Geometry: final body of the model. Coordinates: model frame, mm. Face numbers are marked on the shaded views. Round coordinates to 2 decimals unless told otherwise and drop trailing zeros. Loops run counter-clockwise (first coordinate to the right, second up) from the corner with the lowest first, then second, coordinate; pieces in that order, holes last. Notation, with made-up numbers: (14.25, 15) - (38.25, 15) arc R19 ccw to (38.25, 46) - close; hole circle Ø9 at (20, -3.75). An arc over 180 degrees is marked (long way). Answer in a Markdown table with one row per item. Add a question column.
from build123d import *

# Parameters (mm, degrees)
SKETCH_1_R          = 11
SKETCH_1_R_2        = 9.5
EXTRUDE_1_DEPTH     = 82
SKETCH_4_R          = 10
CUT_EXTRUDE_2_DEPTH = 2
CUT_EXTRUDE_START   = -2
SKETCH_5_R          = 10
CUT_EXTRUDE_3_DEPTH = 2
SKETCH_6_R          = 11.5
SKETCH_6_R_2        = 10.5
CUT_EXTRUDE_4_DEPTH = 0.5
SKETCH_7_R          = 11.5
SKETCH_7_R_2        = 10.5
CUT_EXTRUDE_5_DEPTH = 0.5


with BuildPart() as part:
    # Эскиз1 → Бобышка-Вытянуть1 (new body)
    with BuildSketch(Plane.XY):
        Circle(SKETCH_1_R)
        Circle(SKETCH_1_R_2, mode=Mode.SUBTRACT)
    extrude(amount=EXTRUDE_1_DEPTH)

    # Эскиз4 → Вырез-Вытянуть2 (cut)
    with BuildSketch(Plane(origin=(0, 0, 0), x_dir=(-1, 0, 0), z_dir=(0, 0, -1))):
        Circle(SKETCH_4_R)
    extrude(amount=-CUT_EXTRUDE_2_DEPTH, mode=Mode.SUBTRACT)

    # Эскиз5 → Вырез-Вытянуть3 (cut)
    with BuildSketch(Plane.XY.offset(82).offset(CUT_EXTRUDE_START)):
        with Locations(Location((0, 0, 0), (0, 0, 180))):
            Circle(SKETCH_5_R)
    extrude(amount=CUT_EXTRUDE_3_DEPTH, mode=Mode.SUBTRACT)

    # Эскиз6 → Вырез-Вытянуть4 (cut)
    with BuildSketch(Plane.XY.offset(74.5)):
        Circle(SKETCH_6_R)
        Circle(SKETCH_6_R_2, mode=Mode.SUBTRACT)
    cut_extrude_4 = extrude(amount=-CUT_EXTRUDE_4_DEPTH, mode=Mode.SUBTRACT)

    # Эскиз7 → Вырез-Вытянуть5 (cut)
    with BuildSketch(Plane.XY.offset(72)):
        Circle(SKETCH_7_R)
        Circle(SKETCH_7_R_2, mode=Mode.SUBTRACT)
    cut_extrude_5 = extrude(amount=-CUT_EXTRUDE_5_DEPTH, mode=Mode.SUBTRACT)

    # Зеркальное отражение1: Вырез-Вытянуть4, Вырез-Вытянуть5 across plane
    add(cut_extrude_4.mirror(Plane.XY.offset(41)), mode=Mode.SUBTRACT)
    add(cut_extrude_5.mirror(Plane.XY.offset(41)), mode=Mode.SUBTRACT)


solid = part.part
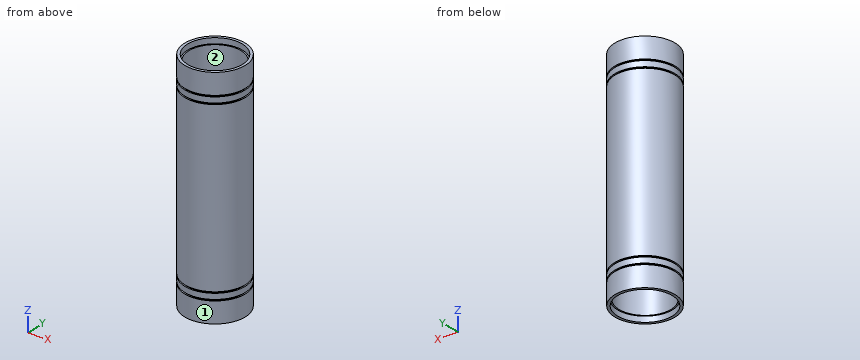
1) Material intervals for line 1 along Y through (x, z) = (0, 9); line 2 along Y through (x, z) = (0, 81.5); line 3 along X through (y, z) = (-0.5, 40), sorted ascending. Write a range as from..to.
2) Pull-direction query (Y, two-part tool) for the marked faces 1 and 2; classes: pulls with the +Y half, pulls with the -Y half, needs draft (parallel to the pull), parting line crosses it, or undercut.
3) Contact query for flat-ended pins moving along their axis: pin 1 Ø1 at (x, z) = (9, 11) entering from -Y; pin 2 Ø1 at (x, z) = (1.5, 26.5) entering from +Y. Output: stop coordinate, or through.
4) Section A-A, the plane z = 12. Return the cut outline in (x, y), and give its area (3 significant figures).
Evaluation:
| question | item | result |
|---|---|---|
| 1 | line 1 | y = -11..-9.5, 9.5..11 |
| 1 | line 2 | y = -11..-10, 10..11 |
| 1 | line 3 | x = -10.99..-9.49, 9.49..10.99 |
| 2 | face 1 | parting line crosses it |
| 2 | face 2 | undercut |
| 3 | pin 1 | stops at y = -6.98 |
| 3 | pin 2 | stops at y = 10.95 |
| 4 | outline | circle Ø22 at (0, 0); hole circle Ø19 at (0, 0) |
| 4 | area | 96.6 mm² |
